```python
from build123d import *

# Parameters (mm, degrees)
SKETCH019_W      = 8.5
SKETCH019_H      = 90
EXTRUDE015_DEPTH = 5
SKETCH020_R      = 1.6
HOLE006_DEPTH    = 5
HOLE006_TIPS_R   = 1.6


with BuildPart() as part:
    # Sketch019 (on Face9 of BaseFeature002) → Extrude015 (new body)
    with BuildSketch(Plane.XY):
        with Locations((69.820944, 71.605001)):
            Rectangle(SKETCH019_W, SKETCH019_H)
    extrude(amount=-EXTRUDE015_DEPTH)

    # Sketch020 (on Face5 of Extrude015) → Hole006 (cut)
    with BuildSketch(Plane.XY):
        with Locations((69.800003, 112.380005)):
            Circle(SKETCH020_R)
        with Locations((69.799998, 73.219998)):
            Circle(SKETCH020_R)
        with Locations((69.799998, 30.879999)):
            Circle(SKETCH020_R)
    extrude(amount=-HOLE006_DEPTH, mode=Mode.SUBTRACT)

    # Hole006 tips → Hole006 tip 1 section 0
    with BuildSketch(Plane.XY.offset(-5), mode=Mode.PRIVATE) as hole006_tip_1_s0:
        with Locations((69.800003, 112.380005)):
            Circle(HOLE006_TIPS_R)
    loft([hole006_tip_1_s0.sketch, Vertex(69.800003, 112.380005, -5.961377)], mode=Mode.SUBTRACT)

    # Hole006 tips → Hole006 tip 2 section 0
    with BuildSketch(Plane.XY.offset(-5), mode=Mode.PRIVATE) as hole006_tip_2_s0:
        with Locations((69.799998, 73.219998)):
            Circle(HOLE006_TIPS_R)
    loft([hole006_tip_2_s0.sketch, Vertex(69.799998, 73.219998, -5.961377)], mode=Mode.SUBTRACT)

    # Hole006 tips → Hole006 tip 3 section 0
    with BuildSketch(Plane.XY.offset(-5), mode=Mode.PRIVATE) as hole006_tip_3_s0:
        with Locations((69.799998, 30.879999)):
            Circle(HOLE006_TIPS_R)
    loft([hole006_tip_3_s0.sketch, Vertex(69.799998, 30.879999, -5.961377)], mode=Mode.SUBTRACT)


solid = part.part
```
Model file for the job. Use its own axes, mm. Round coordinates to 2 decimals unless told otherwise and drop trailing zeros. Write each loop counter-clockwise with the first axis right and the second up, starting at its lowest first coordinate (ties: lowest second). Pieces come first, ordered by that corner, then holes. Notation, with made-up numbers: M 0.5,24 L 17.5,24 A32 ccw 17.5,51 Z; hole C 36.25,2.25 d9. An arc over 180 degrees is marked long. Put each result on its own line as item: value.
Item 1: Flat gauge pin, fed straight in: P1, Ø3, axis at x = 69.8, y = 112.38, coming from the -Z side. Where does the tip first touch, or does it go through?
Responses:
P1: through
Item 2: Mould opens along Y. For faces 1 (the cylindrical face through (71.28, 72.61, -2.46)), 2 (the flat face through (72, 72, -5)), 3 (the flat face through (70, 116.605, -2)) say: +Y half, -Y half, draft (parallel to the pull), parting line (faces both ways), or undercut.
Responses:
face 1: undercut
face 2: draft
face 3: +Y half
Item 3: Cut at A-A (y = 30.88). List the corners of the cut face in (x, z).
Responses:
outline: M 65.57,-5 L 68.2,-5 L 68.2,0 L 65.57,0 Z; M 71.4,-5 L 74.07,-5 L 74.07,0 L 71.4,0 Z
Item 4: Probe L1, parallel to Y at x = 70, z = -2.5 (3 decimals); L2, parallel to X at y = 30.88, z = -2.35; L3, parallel to Y at x = 71, z = -1.35 (3 decimals). List the from-to ranges inside material, lowest first. Write a range as from..to.
Responses:
L1: 26.605..29.293, 32.467..71.633, 74.807..110.793, 113.967..116.605
L2: 65.57..68.2, 71.4..74.07
L3: 26.605..29.822, 31.938..72.162, 74.278..111.322, 113.438..116.605
Item 5: Cut at B-B (z = -1.25). List the corners of the cut face in (x, y) (3 decimals).
Responses:
outline: M 65.571,26.605 L 74.071,26.605 L 74.071,116.605 L 65.571,116.605 Z; hole C 69.8,30.88 d3.2; hole C 69.8,73.22 d3.2; hole C 69.8,112.38 d3.2
Item 6: Cut at C-C (x = 69). List the corners of the cut face in (y, z) (3 decimals).
Responses:
outline: M 26.605,-5 L 29.494,-5 L 29.494,0 L 26.605,0 Z; M 32.266,-5 L 71.834,-5 L 71.834,0 L 32.266,0 Z; M 74.606,-5 L 110.994,-5 L 110.994,0 L 74.606,0 Z; M 113.766,-5 L 116.605,-5 L 116.605,0 L 113.766,0 Z
